Geometry: final body of the model. Coordinates: model frame, mm. A direction names the side the tool comes from. Give positions to 0.01 mm unless a question says otherwise; leave off trailing zeros. Loops run counter-clockwise (first coordinate to the right, second up) from the corner with the lowest first, then second, coordinate; pieces in that order, holes last. Notation, with made-up numbers: (-31, 76.5) - (16, 76.5) arc R11 ccw to (16, 93.5) - close; hole circle Ø6 at (-10, 72.5). An arc over 180 degrees is marked (long way). Answer in a Markdown table with one row per item.
from build123d import *

# Parameters (mm, degrees)
F0_W     = 30
F0_H     = 30
F1_DEPTH = 2
F2_W     = 22
F2_H     = 22
F2_W_2   = 18
F2_H_2   = 18
F3_DEPTH = 10
F4_W     = 22
F4_H     = 22
F4_W_2   = 2
F4_H_2   = 12
F4_W_3   = 14
F4_H_3   = 2
F4_W_4   = 13
F5_DEPTH = 2
F6_R     = 1.99999
F7_W     = 12.5
F7_H     = 5
F7_W_2   = 5
F7_H_2   = 12.5
F8_DEPTH = 12


# Not quite as in the source:
# - a fillet or chamfer is up to 0.001 mm smaller than in the source, because OpenCascade refuses the exact size


with BuildPart() as f1:
    # F0 (on Top) → F1 (new body)
    with BuildSketch(Plane.XY):
        with Locations((15, -15)):
            Rectangle(F0_W, F0_H)
    extrude(amount=F1_DEPTH)

    # F2 (on face) → F3 (join)
    with BuildSketch(Plane.XY.offset(2)):
        with Locations((19, -19)):
            Rectangle(F2_W, F2_H)
        with Locations((19, -19)):
            Rectangle(F2_W_2, F2_H_2, mode=Mode.SUBTRACT)
    extrude(amount=F3_DEPTH)

    # F4 (on face) → F5 (join)
    with BuildSketch(Plane.XY.offset(12)):
        with Locations((19, -19)):
            Rectangle(F4_W, F4_H)
        Polygon((13, -28), (10, -28), (10, -25), (10, -13), (10, -10), (12, -10), (26, -10), (28, -10), (28, -13), (28, -25), (28, -28), (26, -28), align=None, mode=Mode.SUBTRACT)
        with Locations((11, -19)):
            Rectangle(F4_W_2, F4_H_2)
        with Locations((19, -11)):
            Rectangle(F4_W_3, F4_H_3)
        with Locations((27, -19)):
            Rectangle(F4_W_2, F4_H_2)
        with Locations((19.5, -27)):
            Rectangle(F4_W_4, F4_H_3)
    extrude(amount=F5_DEPTH)

    # F6 (radius 2 in the source; OpenCascade refuses exactly that, so slightly less here)
    f6_edges = [f1.edges().sort_by_distance(p)[0] for p in [
        (10, -19, 12),
        (28, -19, 12),
        (19, -10, 12),
        (19.5, -28, 12),
    ]]
    fillet(f6_edges, radius=F6_R)

    # F7 (on face) → F8 (cut, through all)
    with BuildSketch(Plane.XY.offset(14)):
        with Locations((27.75, -19)):
            Rectangle(F7_W, F7_H)
        with Locations((19, -27.75)):
            Rectangle(F7_W_2, F7_H_2)
        with Locations((19, -19)):
            Rectangle(F7_W_2, F7_H)
        with Locations((10.25, -19)):
            Rectangle(F7_W, F7_H)
        with Locations((19, -10.25)):
            Rectangle(F7_W_2, F7_H_2)
    extrude(amount=-F8_DEPTH, mode=Mode.SUBTRACT)


solid = f1.part
Q1. Material intervals for line 1 along Y through (x, z) = (11.5, 3.25); line 2 along X through (y, z) = (-14.5, 4.5); line 3 along X through (y, z) = (-8.25, 13.5), sorted ascending.
Check values:
| item | result |
|---|---|
| line 1 | -30 to -28, -10 to -8 |
| line 2 | 8 to 10, 28 to 30 |
| line 3 | 8 to 16.5, 21.5 to 30 |
Q2. Draft query along Y for faces 5 (the flat face through (26, -11, 13)), 6 (the flat face through (12, -8, 8)), 7 (the cylindrical face through (10.6, -14.73, 11.43)), 8 (the flat face through (8, -12, 8)). Return one class per face: pulls with the +Y half, pulls with the -Y half, needs draft (parallel to the pull), parting line crosses it, or undercut.
Check values:
| item | result |
|---|---|
| face 5 | undercut |
| face 6 | pulls with the +Y half |
| face 7 | undercut |
| face 8 | needs draft |
Q3. Reachability of faces 1 (the flat face through (28.5, -16.5, 9.4)), 2 (the flat face through (25, -28, 7)), 3 (the flat face through (11, -25, 13)), 4 (the flat face through (16.5, -9.6, 9.4)) from +Z, -Z, +X, -X, +Y, -Y: full face, straight path, thin tool, end or side. Return the list, or none.
Check values:
| item | result |
|---|---|
| face 1 | +Z, +X, -X |
| face 2 | none |
| face 3 | +Z |
| face 4 | +Z, +Y, -Y |
Q4. Cut plane B-B (x = 26.5). Output: boundary loops of the cut face in (y, z).
Check values:
| item | result |
|---|---|
| outline | (-30, 0) - (0, 0) - (0, 2) - (-8, 2) - (-8, 14) - (-10, 14) - (-10, 2) - (-28, 2) - (-28, 14) - (-30, 14) - close; (-25, 11.94) - (-21.5, 11.94) - (-21.5, 14) - (-25, 14) - close; (-16.5, 11.94) - (-13, 11.94) - (-13, 14) - (-16.5, 14) - close |
Q5. Cut plane C-C (y = -8.75). Output: boundary loops of the cut face in (x, z).
Check values:
| item | result |
|---|---|
| outline | (0, 0) - (30, 0) - (30, 14) - (21.5, 14) - (21.5, 2) - (16.5, 2) - (16.5, 14) - (8, 14) - (8, 2) - (0, 2) - close |
Q6. First-contact query: pin 1 (3 mm diameter, centred on x = 19, y = -13.5, fed in from +Z); pin 2 (5 mm diameter, centred on y = -16, z = 5.5, fed in from -X); pin 3 (8 mm diameter, centred on x = 23.5, z = 11, fed in from +Y); pin 4 (12 mm diameter, centred on x = 13, y = -15.5, fed in from +Z). Flat tips, straight axial feed; report the tip coordinate or a pass-through.
Check values:
| item | result |
|---|---|
| pin 1 | z = 2 |
| pin 2 | x = 8 |
| pin 3 | y = -8 |
| pin 4 | z = 14 |
Q7. Cut plane D-D (x = 5.75). Output: boundary loops of the cut face in (y, z), and give its area (3 significant figures).
Check values:
| item | result |
|---|---|
| outline | (-30, 0) - (0, 0) - (0, 2) - (-30, 2) - close |
| area | 60.0 mm² |
Q8. Cut plane A-A (z = 7.5). Output: boundary loops of the cut face in (x, y).
Check values:
| item | result |
|---|---|
| outline | (8, -30) - (16.5, -30) - (16.5, -28) - (10, -28) - (10, -21.5) - (8, -21.5) - close; (8, -16.5) - (10, -16.5) - (10, -10) - (16.5, -10) - (16.5, -8) - (8, -8) - close; (21.5, -30) - (30, -30) - (30, -21.5) - (28, -21.5) - (28, -28) - (21.5, -28) - close; (21.5, -10) - (28, -10) - (28, -16.5) - (30, -16.5) - (30, -8) - (21.5, -8) - close |
